Autodesk Inventor part; units mm, degrees
ref_plane "YZ Plane" through (0, 0, 0) normal (1, 0, 0) x (0, 1, 0)
ref_plane "XZ Plane" through (0, 0, 0) normal (0, 1, 0) x (-1, 0, 0)
ref_plane "XY Plane" through (0, 0, 0) normal (0, 0, 1) x (1, 0, 0)
sketch "Skizze1" plane through (0, 0, 0) normal (1, 0, 0) x (0, 1, 0)
  circle A0 centre (0, 0) radius 20
  dimension "d0" = 40
extrude "Extrusion1" add sketch "Skizze1" along normal blind 1
sketch "Skizze2" plane through (1, 0, 0) normal (1, 0, 0) x (0, 0, -1)
  circle A0 centre (0, 0) radius 20
  circle A1 centre (0, 0) radius 17
  dimension "d3" = 34
extrude "Extrusion2" add sketch "Skizze2" along normal blind 20 contours A1
sketch "Skizze5" plane through (0, 0, 0) normal (-1, 0, 0) x (0, 0, 1)
  circle A0 centre (0, 0) radius 20
  circle A1 centre (0, 0) radius 5
  dimension "d12" = 10
extrude "Extrusion5" add sketch "Skizze5" along normal blind 10 contours A1
sketch "Skizze6" plane through (21, 0, 0) normal (1, 0, 0) x (0, 0, -1)
  circle A0 centre (0, 0) radius 17
  circle A1 centre (0, 0) radius 11
  dimension "d15" = 22
extrude "Extrusion6" cut sketch "Skizze6" against normal through all contours A1
properties part number "Rolle_schieber" material "PC/ABS-Kunststoff"
Read the model definition and answer for the solid it produces. Units are mm, in the model's axes. A direction names the side the tool comes from. Coordinates: 2 decimals unless noted, no trailing zeros. Write each loop counter-clockwise with the first axis right and the second up, starting at its lowest first coordinate (ties: lowest second). Pieces come first, ordered by that corner, then holes. Notation, with made-up numbers: (62, -5.75) - (106, -5.75) arc R15 ccw to (106, 17.25) - close; hole circle Ø4 at (82, -28.75). An arc over 180 degrees is marked (long way). Answer as a JSON object with one key per item and string values. Group by question number.
1. A cutting plane is placed at A-A (z = 0). Determine the outline of the cut face in (x, y), plus the area to 3 significant figures.
2. Which of the six approach directions +Z, -Z, +X, -X, +Y, -Y give full straight-line access (tool end or side, diameter ignored) to faces 4 (the cylindrical face through (10.86, -14.334, -9.139)), 5 (the flat face through (0, 9, -9))?
3. A cutting plane is placed at C-C (x = 18). Determine the outline of the cut face in (y, z), plus the area to 3 significant figures.
4. Each of these flat-tipped pins is pushed along its axis until it touches: P1, Ø2, axis at x = 6.5, z = -11.5, coming from the +Y side; P2, Ø2, axis at x = 5, z = 5, coming from the -Y side; P3, Ø6, axis at x = 5, z = -8.5, coming from the +Y side. Where does it stop, or does it pass through?
5. Consider L1, parallel to Y at x = 16.5, z = 0; L2, parallel to Z at x = 3.75, y = 9; L3, parallel to Y at x = 11.5, z = 3. Determine where each line is inside the solid, lowest interval first. Write a range as [from, to].
6. The mould has two halves that part along Y. Classify faces 1 (the cylindrical face through (0.493, -4.336, 19.524)), 2 (the flat face through (21, -11, -4)), 3 (the cylindrical face through (10.65, -10.74, 2.38)): +Y half, -Y half, draft (parallel to the pull), parting line (faces both ways), or undercut.
7. A cutting plane is placed at B-B (y = 7). Determine the outline of the cut face in (x, z) (3 decimals).
8. A cutting plane is placed at D-D (z = -15). Determine the outline of the cut face in (x, y).
Worked out:
{
 "1": {"outline": "(0, -20) - (1, -20) - (1, -17) - (21, -17) - (21, -11) - (0, -11) - close; (0, 11) - (21, 11) - (21, 17) - (1, 17) - (1, 20) - (0, 20) - close", "area": "258 mm²"},
 "2": {"face 4": "+X", "face 5": "+Z, -Z, -X, +Y, -Y"},
 "3": {"outline": "circle Ø34 at (0, 0); hole circle Ø22 at (0, 0)", "area": "528 mm²"},
 "4": {"P1": "stops at y = 13.37", "P2": "stops at y = -16.52", "P3": "stops at y = 16.09"},
 "5": {"L1": "y = [-17, -11], [11, 17]", "L2": "z = [-14.42, -6.32], [6.32, 14.42]", "L3": "y = [-16.73, -10.58], [10.58, 16.73]"},
 "6": {"face 1": "parting line", "face 2": "draft", "face 3": "undercut"},
 "7": {"outline": "(0, -18.735) - (1, -18.735) - (1, -15.492) - (21, -15.492) - (21, -8.485) - (0, -8.485) - close; (0, 8.485) - (21, 8.485) - (21, 15.492) - (1, 15.492) - (1, 18.735) - (0, 18.735) - close"},
 "8": {"outline": "(0, -13.23) - (1, -13.23) - (1, -8) - (21, -8) - (21, 8) - (1, 8) - (1, 13.23) - (0, 13.23) - close"}
}
